Model file for the job. Use its own axes, mm. A direction names the side the tool comes from. Round coordinates to 2 decimals unless told otherwise and drop trailing zeros. Write each loop counter-clockwise with the first axis right and the second up, starting at its lowest first coordinate (ties: lowest second). Pieces come first, ordered by that corner, then holes.
```python
from build123d import *

# Parameters (mm, degrees)
MODEL_R                  = 7.35
MODEL_R_2                = 7.3
MODEL_R_3                = 1.85
RESSALTO_EXTRUS_O1_DEPTH = 8
ESBO_O3_R                = 11.3
CORTE_EXTRUS_O1_DEPTH    = 2
ESBO_O4_R                = 11.3
CORTE_EXTRUS_O2_DEPTH    = 2
ESBO_O2_R                = 3.3
CORTE_EXTRUS_O4_DEPTH    = 2
ESBO_O7_W                = 2.8
ESBO_O7_H                = 2.8
CORTE_EXTRUS_O6_DEPTH    = 6
ESBO_O8_W                = 2.8
ESBO_O8_H                = 2.8
CORTE_EXTRUS_O7_DEPTH    = 6
ESBO_O10_W               = 2.8
ESBO_O10_H               = 2.8
CORTE_EXTRUS_O9_DEPTH    = 6
ESBO_O11_R               = 7.65
ESBO_O11_R_2             = 7.35
ESBO_O11_R_3             = 9.65
ESBO_O11_R_4             = 9.35
ESBO_O11_R_5             = 9.6
ESBO_O11_R_6             = 9.3
ESBO_O11_R_7             = 7.6
ESBO_O11_R_8             = 7.3
RESSALTO_EXTRUS_O2_DEPTH = 2
RESSALTO_EXTRUS_O3_DEPTH = 8
ESBO_O6_R                = 1.5
CORTE_EXTRUS_O5_DEPTH    = 10


with BuildPart() as part:
    # Model → Ressalto-extrusão1 (new body)
    with BuildSketch(Plane.XY):
        with BuildLine():
            Line((0, 0), (39, 0))
            Line((39, 0), (39.7, 0))
            Line((39.7, 0), (39.7, -6.854833996))
            Line((39.7, -6.854833996), (52.445166004, -19.6))
            Line((52.445166004, -19.6), (59.445166004, -26.6))
            Line((59.445166004, -26.6), (81.699998871, -26.6))
            ThreePointArc((81.699998871, -26.6), (102.949229032, -12.401719466), (97.963455967, 12.663455967))
            Line((97.963455967, 12.663455967), (63.677897161, 46.949014774))
            Line((63.677897161, 46.949014774), (50.111140335, 46.949014774))
            Line((50.111140335, 46.949014774), (15.50707852, 46.949014774))
            Line((15.50707852, 46.949014774), (0, 31.441936254))
            Line((0, 31.441936254), (0, 0))
        make_face()
        with Locations((59.072583002, 19.027416998)):
            Circle(MODEL_R, mode=Mode.SUBTRACT)
        with Locations((81.7, -3.6)):
            Circle(MODEL_R_2, mode=Mode.SUBTRACT)
        with Locations((6.960594046, 15.730973227)):
            Circle(MODEL_R_3, mode=Mode.SUBTRACT)
        with Locations((6.960594046, 31.230973227)):
            Circle(MODEL_R_3, mode=Mode.SUBTRACT)
        with Locations((20.383987804, 38.980973227)):
            Circle(MODEL_R_3, mode=Mode.SUBTRACT)
        with Locations((33.807381563, 31.230973227)):
            Circle(MODEL_R_3, mode=Mode.SUBTRACT)
        with Locations((33.807381563, 15.730973227)):
            Circle(MODEL_R_3, mode=Mode.SUBTRACT)
        with Locations((20.383987804, 7.980973227)):
            Circle(MODEL_R_3, mode=Mode.SUBTRACT)
        with Locations((27.383987804, 23.480973227)):
            Circle(MODEL_R, mode=Mode.SUBTRACT)
        Polygon((72, -15), (52, 5), (45, 5), (45, -4), (61, -20), (77, -20), align=None, mode=Mode.SUBTRACT)
    extrude(amount=RESSALTO_EXTRUS_O1_DEPTH)

    # Esboço3 → Corte-extrusão1 (cut)
    with BuildSketch(Plane.XY):
        with Locations((81.7, -3.6)):
            Circle(ESBO_O3_R)
        with Locations((59.0726, 19.0274)):
            Circle(ESBO_O3_R)
        with Locations((27.384004802, 23.480956229)):
            Circle(ESBO_O3_R)
    extrude(amount=CORTE_EXTRUS_O1_DEPTH, mode=Mode.SUBTRACT)

    # Esboço4 → Corte-extrusão2 (cut)
    with BuildSketch(Plane.XY.offset(8)):
        with Locations((81.7, -3.6)):
            Circle(ESBO_O4_R)
        with Locations((59.0726, 19.0274)):
            Circle(ESBO_O4_R)
        with Locations((27.384004802, 23.480956229)):
            Circle(ESBO_O4_R)
    extrude(amount=-CORTE_EXTRUS_O2_DEPTH, mode=Mode.SUBTRACT)

    # Esboço2 → Corte-extrusão4 (cut)
    with BuildSketch(Plane.XY):
        with Locations((6.960594802, 15.730956229)):
            Circle(ESBO_O2_R)
        with Locations((6.960594802, 31.230956229)):
            Circle(ESBO_O2_R)
        with Locations((33.807404802, 15.730956229)):
            Circle(ESBO_O2_R)
        with Locations((20.384004802, 38.980956229)):
            Circle(ESBO_O2_R)
        with Locations((33.807404802, 31.230956229)):
            Circle(ESBO_O2_R)
        with Locations((20.384004802, 7.980976229)):
            Circle(ESBO_O2_R)
    extrude(amount=CORTE_EXTRUS_O4_DEPTH, mode=Mode.SUBTRACT)

    # Esboço7 → Corte-extrusão6 (cut)
    with BuildSketch(Plane(origin=(55.313455967, 55.313455967, 0), x_dir=(0, 0, -1), z_dir=(0.7071067811865474, 0.7071067811865477, 0))):
        with Locations((-4, -52.072657306)):
            Rectangle(ESBO_O7_W, ESBO_O7_H)
        with Locations((-4, -20.072657306)):
            Rectangle(ESBO_O7_W, ESBO_O7_H)
    extrude(amount=-CORTE_EXTRUS_O6_DEPTH, mode=Mode.SUBTRACT)

    # Esboço8 → Corte-extrusão7 (cut)
    with BuildSketch(Plane(origin=(0, 46.949014774, 0), x_dir=(1, 0, 0), z_dir=(0, 1, 0))):
        with Locations((39.59248784, -4)):
            Rectangle(ESBO_O8_W, ESBO_O8_H)
    extrude(amount=-CORTE_EXTRUS_O7_DEPTH, mode=Mode.SUBTRACT)

    # Esboço10 → Corte-extrusão9 (cut)
    with BuildSketch(Plane(origin=(16.422583002, 16.422583002, 0), x_dir=(0, 0, 1), z_dir=(-0.7071067811865477, -0.7071067811865475, 0))):
        with Locations((4, -46.881179593)):
            Rectangle(ESBO_O10_W, ESBO_O10_H)
    extrude(amount=-CORTE_EXTRUS_O9_DEPTH, mode=Mode.SUBTRACT)

    # Esboço11 → Ressalto-extrusão2 (add)
    with BuildSketch(Plane.XY.offset(6)):
        with BuildLine():
            ThreePointArc((34.519218365, 29.523405258), (36.162851789, 26.698743748), (36.733987804, 23.480973227))
            ThreePointArc((36.733987804, 23.480973227), (36.162851789, 20.263202705), (34.519218365, 17.438541195))
            ThreePointArc((34.519218365, 17.438541195), (34.658656459, 17.373480777), (34.792205686, 17.297057977))
            ThreePointArc((34.792205686, 17.297057977), (36.456247792, 20.192113437), (37.033987804, 23.480973227))
            ThreePointArc((37.033987804, 23.480973227), (36.456247792, 26.769833017), (34.792205686, 29.664888476))
            ThreePointArc((34.792205686, 29.664888476), (34.658656459, 29.588465677), (34.519218365, 29.523405258))
        make_face()
        with BuildLine():
            ThreePointArc((31.997376327, 15.348375466), (18.033987804, 23.480973227), (31.997376327, 31.613570987))
            ThreePointArc((31.997376327, 31.613570987), (32.03543104, 31.762660488), (32.085743581, 31.908071934))
            ThreePointArc((32.085743581, 31.908071934), (17.733987804, 23.480973227), (32.085743581, 15.05387452))
            ThreePointArc((32.085743581, 15.05387452), (32.03543104, 15.199285965), (31.997376327, 15.348375466))
        make_face()
        with Locations((27.383987804, 23.480973227)):
            Circle(ESBO_O11_R)
        with Locations((27.383987804, 23.480973227)):
            Circle(ESBO_O11_R_2, mode=Mode.SUBTRACT)
        with Locations((59.072583002, 19.027416998)):
            Circle(ESBO_O11_R_3)
        with Locations((59.072583002, 19.027416998)):
            Circle(ESBO_O11_R_4, mode=Mode.SUBTRACT)
        with Locations((59.072583002, 19.027416998)):
            Circle(ESBO_O11_R)
        with Locations((59.072583002, 19.027416998)):
            Circle(ESBO_O11_R_2, mode=Mode.SUBTRACT)
        with Locations((81.7, -3.6)):
            Circle(ESBO_O11_R_5)
        with Locations((81.7, -3.6)):
            Circle(ESBO_O11_R_6, mode=Mode.SUBTRACT)
        with Locations((81.7, -3.6)):
            Circle(ESBO_O11_R_7)
        with Locations((81.7, -3.6)):
            Circle(ESBO_O11_R_8, mode=Mode.SUBTRACT)
    extrude(amount=RESSALTO_EXTRUS_O2_DEPTH)

    # Esboço13 → Ressalto-extrusão3 (add)
    with BuildSketch(Plane.XY.offset(8)):
        Polygon((0, 31.441936254), (-20, 11.441936254), (-20, 0), (0, 0), align=None)
    extrude(amount=-RESSALTO_EXTRUS_O3_DEPTH)

    # Esboço6 → Corte-extrusão5 (cut)
    with BuildSketch(Plane.XZ):
        with Locations(Location((4.7, 4, 0), (0, 0, 270))):
            Circle(ESBO_O6_R)
        with Locations(Location((23.7, 4, 0), (0, 0, 270))):
            Circle(ESBO_O6_R)
        with Locations(Location((-14.3, 4, 0), (0, 0, 270))):
            Circle(ESBO_O6_R)
    extrude(amount=-CORTE_EXTRUS_O5_DEPTH, mode=Mode.SUBTRACT)


solid = part.part
```
1) Cut at D-D on x = 95.5. List the corners of the cut face in (y, z), and give its area (3 significant figures).
2) Cut at B-B on x = -14.3. List the corners of the cut face in (y, z).
3) Wall check: probe 1 along Y at (x, z) = (84, 7.75); probe 2 along X at (y, z) = (6, 1.5); probe 3 along Y at (x, z) = (67, 7.5). Give the ranges that are in metal, low to high.
4) Flat gauge pins, fed straight in: pin 1 Ø9.5 at (x, y) = (58.5, 21) entering from +Z; pin 2 Ø3 at (y, z) = (4.5, 1) entering from +X; pin 3 Ø3.5 at (x, z) = (4.7, 4) entering from -Y; pin 4 Ø2.5 at (y, z) = (-1, 4.5) entering from +X. Where does each tip first touch, or does it go through?
5) Cut at A-A on x = 30. List the corners of the cut face in (y, z).
6) Cut at C-C on y = 25. Give the number of separate pieces and of enclosed holes in the cut face, and give its area (3 significant figures).
7) Pull direction X, two halves, no side cores. Call faces 5 (the face through (-20, 6, 4)), 6 (the face through (102.8, -12.75, 3.94)), 7 (the face through (70, -26.6, 4)), 8 (the face through (38.683, 23.362, 7.014)): released by +X, released by -X, zero draft, split by the parting line, or undercut.
8) Which spindle directions (+Z, -Z, +X, -X, +Y, -Y) get a long thin tool onto all of the face, cutting with end or side? Do faces 1 (the face through (19.74, 23.82, 6.99)), 2 (the face through (51.73, 19.35, 4.96)), 3 (the face through (66.425, 40.018, 4.02)), 4 (the face through (35.96, 33.73, 0.99)). Say none if no direction does.
Result sheet:
1. outline: (-22, 0) - (15.13, 0) - (15.13, 8) - (-22, 8) - close
1. area: 297 mm2
2. outline: (0, 0) - (17.14, 0) - (17.14, 8) - (0, 8) - (0, 5.5) - (10, 5.5) - (10, 2.5) - (0, 2.5) - close
3. probe 1: y = -26.48 to -14.66, -12.92 to -12.61, -10.84 to -10.53, 3.33 to 3.64, 5.41 to 5.72, 7.46 to 26.63
3. probe 2: x = -20 to 17.74, 23.02 to 75.74, 87.66 to 102.6
3. probe 3: y = -26.6 to -20, -10 to 10.97, 13.52 to 14.07, 23.99 to 24.53, 27.08 to 43.63
4. pin 1: passes through
4. pin 2: stops at x = 103.73
4. pin 3: stops at y = 0
4. pin 4: stops at x = 104.66
5. outline: (0, 0) - (12.49, 0) - (12.49, 2) - (16.61, 2) - (16.61, 8) - (16.29, 8) - (16.29, 6) - (14.5, 6) - (14.5, 8) - (14.19, 8) - (14.19, 6) - (12.49, 6) - (12.49, 8) - (0, 8) - close; (30.35, 2) - (34.47, 2) - (34.47, 0) - (46.95, 0) - (46.95, 8) - (34.47, 8) - (34.47, 6) - (32.77, 6) - (32.77, 8) - (32.46, 8) - (32.46, 6) - (30.67, 6) - (30.67, 8) - (30.35, 8) - close
6. separate pieces: 3
6. enclosed holes: 0
6. area: 484 mm2
7. face 5: released by -X
7. face 6: released by +X
7. face 7: zero draft
7. face 8: undercut
8. face 1: +Z
8. face 2: +Z, -Z
8. face 3: none
8. face 4: -Z
